Check sheet for the modelled part. Datum: model origin and axes. Units: mm. Face numbers are marked on the shaded views. A direction names the side the tool comes from. Give positions to 0.01 mm unless a question says otherwise; leave off trailing zeros. Loops run counter-clockwise (first coordinate to the right, second up) from the corner with the lowest first, then second, coordinate; pieces in that order, holes last. Notation, with made-up numbers: (11, 37.25) -> (51, 37.25) arc R14 cw to (51, 61.25) -> close; hole circle Ø3 at (23.5, 36). An arc over 180 degrees is marked (long way). Answer as CSV lines item,"result". Start each with the question number.
(1) Access from +Z, -Z, +X, -X, +Y, -Y to the whole of each face (thin tool, end or side, straight path). Record for the marked faces 1, 2 and 3.
(2) Material ranges on line 1 (X direction, y = -7.75, z = 21); line 2 (X direction, y = -9.5, z = 18) (3 decimals), recorded low to high. Write a range as from..to.
(3) Section check A-A on z = 32. Enter the section's corners in (x, y) (3 decimals).
(4) Gauge pin test, flat ends, axial feed: pin 1 Ø3 at (x, z) = (6.5, 29.5) entering from -Y; pin 2 Ø2 at (y, z) = (-10, 34) entering from -X (3 decimals); pin 3 Ø4 at (x, z) = (4.826, 20.955) entering from -Y; pin 4 Ø4 at (y, z) = (-7.5, 19) entering from -X. Record the tip position at first contact, or that the pin passes through.
(5) Section check C-C on y = -12.25. Enter the section's corners in (x, z) (3 decimals), plus the area to 3 significant figures.
(6) Section check B-B on z = 20. Enter the section's corners in (x, y) (3 decimals), plus the area to 3 significant figures.
from build123d import *

# Parameters (mm, degrees)
BOSS_EXTRUDE1_DEPTH    = 41.91
F_10_CLEARANCE_HOLE1_D = 5.1054


with BuildPart() as part:
    # Sketch1 → Boss-Extrude1 (new body)
    with BuildSketch(Plane.XY):
        Polygon((0, 0), (114.3, 0), (114.3, -8.89), (104.775, -8.89), (104.775, -15.24), (9.525, -15.24), (9.525, -8.89), (0, -8.89), align=None)
    extrude(amount=BOSS_EXTRUDE1_DEPTH)

    # #10 Clearance Hole1 (through all)
    with Locations(Plane(origin=(4.826, 0, 20.955), x_dir=(0, 0, 1), z_dir=(0, 1, 0))):
        with Locations((0, 0), (0, 104.648)):
            Hole(F_10_CLEARANCE_HOLE1_D / 2)


solid = part.part
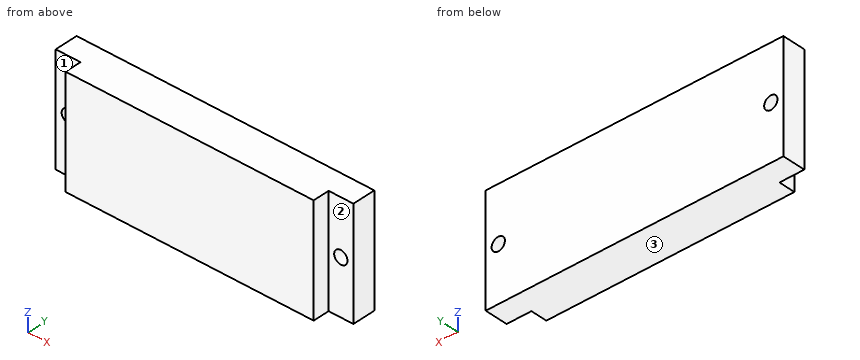
Working result:
1,face 1,"+Z, -Z, -X, -Y"
1,face 2,"+Z, -Z, +X, -Y"
1,face 3,"-Z, +X, -X, +Y, -Y"
2,line 1,"x = 0..2.27, 7.38..106.92, 112.03..114.3"
2,line 2,"x = 9.525..104.775"
3,outline,"(0, -8.89) -> (9.525, -8.89) -> (9.525, -15.24) -> (104.775, -15.24) -> (104.775, -8.89) -> (114.3, -8.89) -> (114.3, 0) -> (0, 0) -> close"
4,pin 1,"stops at y = -8.89"
4,pin 2,"stops at x = 9.525"
4,pin 3,"passes through"
4,pin 4,"stops at x = 0"
5,outline,"(9.525, 0) -> (104.775, 0) -> (104.775, 41.91) -> (9.525, 41.91) -> close"
5,area,"3,990 mm^2"
6,outline,"(0, -8.89) -> (2.459, -8.89) -> (2.459, 0) -> (0, 0) -> close; (7.193, -8.89) -> (9.525, -8.89) -> (9.525, -15.24) -> (104.775, -15.24) -> (104.775, -8.89) -> (107.107, -8.89) -> (107.107, 0) -> (7.193, 0) -> close; (111.841, -8.89) -> (114.3, -8.89) -> (114.3, 0) -> (111.841, 0) -> close"
6,area,"1,540 mm^2"
